The model under review builds one solid part; all positions refer to its coordinate system, in mm. A direction names the side the tool comes from. Coordinates: 2 decimals unless noted, no trailing zeros. Loops run counter-clockwise (first coordinate to the right, second up) from the corner with the lowest first, then second, coordinate; pieces in that order, holes last. Notation, with made-up numbers: (-29, 35) - (-19, 35) arc R14 cw to (-19, 43) - close; hole circle Ø8 at (81.5, 38.25). An arc over 180 degrees is marked (long way). Use a Markdown table: item, result. Add a question column.
1) Clearance check with flat-ended pins moving along their axes: pin 1 (1 mm diameter, centred on y = -12, z = -29, fed in from -X); pin 2 (3 mm diameter, centred on x = 5, y = -3.5, fed in from +Z); pin 3 (3 mm diameter, centred on x = 8.5, z = -19, fed in from +Y); pin 4 (1.5 mm diameter, centred on x = 2, z = -17.5, fed in from -Y). State where each tip first meets the part, or that it passes through.
2) To check wall thickness, follow L1, parallel to Y at x = 5, z = -9; L2, parallel to Z at x = 6, y = -15.5; L3, parallel to Y at x = 9.25, z = -9. State the ranges of each line that lie inside material, in increasing order. Write a range as [from, to].
3) For faces 4 (the flat face through (5, 1, -38.3)), 5 (the cylindrical face through (0.43, 4.54, -10.05)), 6 (the flat face through (5, -3, -15)), 7 (the flat face through (5, 2, -8)), 8 (the flat face through (5, 4, -32.3)), list the 3-axis set-ups (+Z, -Z, +X, -X, +Y, -Y) from which the entire face can be reached by the end or side of a thin tool; tool diameter is ignored.
4) Add section D-D, the plane y = -20.25. Give the boundary of the cut face in (x, z).
5) Add section B-B, the plane x = 5. Give the boundary of the cut face in (y, z).
6) Add section C-C, the plane z = -21.4. Give the boundary of the cut face in (x, y), and give its area (3 significant figures).
7) Add section A-A, the plane z = -11.4. Give the boundary of the cut face in (x, y).
8) The part is to be moulded in two halves that separate along Y. For faces 1 (the flat face through (5, 0, -41)), 2 (the flat face through (5, 7, -38)), 3 (the flat face through (5, -8, 0)), say which applies: pulls with the +Y half, pulls with the -Y half, needs draft (parallel to the pull), parting line crosses it, or undercut.
```python
from build123d import *

# Parameters (mm, degrees)
F1_DEPTH = 10
F2_R     = 1.35
F3_DEPTH = 15
F4_W     = 15
F4_H     = 42.8
F5_DEPTH = 3
F6_R     = 1.35
F7_DEPTH = 7.001
F8_R     = 1.5


with BuildPart() as f1:
    # F0 (on Right) → F1 (new body)
    with BuildSketch(Plane.YZ):
        Polygon((7, 0), (-23, 0), (-23, -42.8), (0, -42.8), (0, -38.3), (2, -38.3), (2, -42.8), (7, -42.8), (7, -32.3), (0, -32.3), (0, -6), (2, -6), (2, -10.5), (7, -10.5), align=None)
    extrude(amount=F1_DEPTH)

    # F2 (on face) → F3 (cut)
    with BuildSketch(Plane.XY):
        with Locations((5, -3.5)):
            Circle(F2_R)
    extrude(amount=-F3_DEPTH, mode=Mode.SUBTRACT)

    # F4 (on face) → F5 (cut)
    with BuildSketch(Plane(origin=(0, 0, 0), x_dir=(0, -1, 0), z_dir=(-1, 0, 0))):
        with Locations((15.5, -21.4)):
            Rectangle(F4_W, F4_H)
    extrude(amount=-F5_DEPTH, mode=Mode.SUBTRACT)

    # F6 (on face) → F7 (cut, through all)
    with BuildSketch(Plane(origin=(3, 0, 0), x_dir=(0, -1, 0), z_dir=(-1, 0, 0))):
        with Locations((15.5, -21.4)):
            Circle(F6_R)
        with Locations((15.5, -11.4)):
            Circle(F6_R)
        with Locations((15.5, -31.4)):
            Circle(F6_R)
    extrude(amount=-F7_DEPTH, mode=Mode.SUBTRACT)

    # F8
    f8_edges = [f1.edges().sort_by_distance(p)[0] for p in [
        (0, -0.5, 0),
        (10, -8, 0),
        (0, 4.5, -10.5),
        (0, 3.5, -32.3),
        (10, 3.5, -32.3),
        (10, 4.5, -10.5),
        (10, 4.5, -42.8),
        (0, 4.5, -42.8),
    ]]
    fillet(f8_edges, radius=F8_R)


solid = f1.part
```
From the geometry:
| question | item | result |
|---|---|---|
| 1 | pin 1 | stops at x = 3 |
| 1 | pin 2 | stops at z = 0 |
| 1 | pin 3 | stops at y = 0 |
| 1 | pin 4 | stops at y = -8 |
| 2 | L1 | y = [-23, -4.85], [-2.15, 0], [2, 7] |
| 2 | L2 | z = [-42.8, -32.75], [-30.05, -22.75], [-20.05, -12.75], [-10.05, 0] |
| 2 | L3 | y = [-23, 0], [2, 7] |
| 3 | face 4 | -Z, +X, -X |
| 3 | face 5 | -X, +Y |
| 3 | face 6 | +Z |
| 3 | face 7 | +X, -X |
| 3 | face 8 | +X, -X, +Y |
| 4 | outline | (3, -42.8) - (10, -42.8) - (10, -1.5) arc R1.5 ccw to (8.5, 0) - (3, 0) - close |
| 5 | outline | (-23, -42.8) - (0, -42.8) - (0, -38.3) - (2, -38.3) - (2, -42.8) - (7, -42.8) - (7, -32.3) - (0, -32.3) - (0, -6) - (2, -6) - (2, -10.5) - (7, -10.5) - (7, 0) - (-2.15, 0) - (-2.15, -15) - (-4.85, -15) - (-4.85, 0) - (-23, 0) - close; hole circle Ø2.7 at (-15.5, -31.4); hole circle Ø2.7 at (-15.5, -21.4); hole circle Ø2.7 at (-15.5, -11.4) |
| 6 | outline | (0, -8) - (3, -8) - (3, -14.15) - (10, -14.15) - (10, 0) - (0, 0) - close; (3, -23) - (10, -23) - (10, -16.85) - (3, -16.85) - close |
| 6 | area | 166 mm^2 |
| 7 | outline | (0, -8) - (3, -8) - (3, -14.15) - (10, -14.15) - (10, 0) - (0, 0) - close; (3, -23) - (10, -23) - (10, -16.85) - (3, -16.85) - close; hole circle Ø2.7 at (5, -3.5) |
| 8 | face 1 | undercut |
| 8 | face 2 | pulls with the +Y half |
| 8 | face 3 | needs draft |
